Autodesk Inventor part; units mm, degrees
ref_plane "YZ Plane" through (0, 0, 0) normal (1, 0, 0) x (0, 1, 0)
ref_plane "XZ Plane" through (0, 0, 0) normal (0, 1, 0) x (-1, 0, 0)
ref_plane "XY Plane" through (0, 0, 0) normal (0, 0, 1) x (1, 0, 0)
sketch "Sketch1" plane through (0, 0, 0) normal (0, 1, 0) x (-1, 0, 0)
  line L0 (0, -7.0711) -> (0, -142.9289)
  line L1 (7.0711, 0) -> (142.9289, 0)
  line L2 (150, -7.0711) -> (150, -142.9289)
  line L3 (142.9289, -150) -> (7.0711, -150)
  line L4 (139.3934, -10.6066) -> (135.8579, -14.1421)
  line L5 (135.8579, -14.1421) -> (132.3223, -10.6066)
  line L6 (132.3223, -10.6066) -> (135.8579, -14.1421)
  line L7 (135.8579, -14.1421) -> (139.3934, -17.6777)
  line L8 (139.3934, -17.6777) -> (150, -7.0711)
  line L9 (132.3223, -10.6066) -> (142.9289, 0)
  line L10 (139.3934, -139.3934) -> (135.8579, -135.8579)
  line L11 (135.8579, -135.8579) -> (132.3223, -139.3934)
  line L12 (132.3223, -139.3934) -> (142.9289, -150)
  line L13 (135.8579, -135.8579) -> (139.3934, -132.3223)
  line L14 (139.3934, -132.3223) -> (150, -142.9289)
  line L15 (10.6066, -139.3934) -> (14.1421, -135.8579)
  line L16 (14.1421, -135.8579) -> (10.6066, -132.3223)
  line L17 (10.6066, -132.3223) -> (14.1421, -135.8579)
  line L18 (14.1421, -135.8579) -> (17.6777, -139.3934)
  line L19 (17.6777, -139.3934) -> (7.0711, -150)
  line L20 (10.6066, -132.3223) -> (0, -142.9289)
  line L21 (10.6066, -10.6066) -> (14.1421, -14.1421)
  line L22 (14.1421, -14.1421) -> (10.6066, -17.6777)
  line L23 (10.6066, -17.6777) -> (14.1421, -14.1421)
  line L24 (14.1421, -14.1421) -> (17.6777, -10.6066)
  line L25 (7.0711, 0) -> (17.6777, -10.6066)
  line L26 (10.6066, -17.6777) -> (0, -7.0711)
  line L27 (132.3223, -10.6066) -> (75, -67.9289)
  line L28 (67.9289, -75) -> (10.6066, -132.3223)
  line L29 (132.3223, -10.6066) -> (17.6777, -10.6066)
  line L30 (139.3934, -17.6777) -> (139.3934, -132.3223)
  line L31 (132.3223, -139.3934) -> (17.6777, -139.3934)
  line L32 (10.6066, -132.3223) -> (10.6066, -17.6777)
  line L33 (139.3934, -10.6066) -> (135.8579, -14.1421)
  line L34 (14.1421, -135.8579) -> (0, -150)
  line L35 (10.6066, -10.6066) -> (14.1421, -14.1421)
  line L36 (135.8579, -135.8579) -> (139.3934, -139.3934)
  line L37 (139.3934, -132.3223) -> (82.0711, -75)
  line L38 (75, -67.9289) -> (17.6777, -10.6066)
  line L39 (10.6066, -17.6777) -> (67.9289, -75)
  line L40 (75, -82.0711) -> (132.3223, -139.3934)
  line L41 (139.3934, -17.6777) -> (82.0711, -75)
  line L42 (75, -82.0711) -> (17.6777, -139.3934)
  point P0 (0, 0)
  dimension "d0" = 150
extrude "Extrusion1" add sketch "Sketch1" along normal blind 10 contours L26 L32 L20 L0 | L22 L24 L38 L27 L5 L7 L41 L37 L13 L11 L40 L42 L18 L16 L28 L39 | L25 L1 L9 L29 | L31 L12 L3 L19 | L8 L2 L14 L30
sketch "Sketch2" plane through (0, 10, 0) normal (0, 1, 0) x (1, 0, 0)
  line L0 (-17.6777, 10.6066) -> (-27.6777, 10.6066)
  line L1 (-17.6777, 10.6066) -> (-132.3223, 10.6066)
  line L2 (-27.6777, 10.6066) -> (-27.6777, 20.6066)
  line L3 (-75, 67.9289) -> (-17.6777, 10.6066)
  line L4 (-10.6066, 17.6777) -> (-67.9289, 75)
  line L5 (-20.6066, 27.6777) -> (-10.6066, 27.6777)
  line L6 (-10.6066, 27.6777) -> (-10.6066, 17.6777)
  line L7 (-10.6066, 132.3223) -> (-10.6066, 17.6777)
  line L8 (-132.3223, 10.6066) -> (-75, 67.9289)
  line L9 (-132.3223, 10.6066) -> (-122.3223, 10.6066)
  line L10 (-122.3223, 10.6066) -> (-122.3223, 20.6066)
  line L11 (-122.3223, 20.6066) -> (-129.3934, 27.6777)
  line L12 (-82.0711, 75) -> (-139.3934, 17.6777)
  line L13 (-139.3934, 27.6777) -> (-129.3934, 27.6777)
  line L14 (-139.3934, 17.6777) -> (-139.3934, 132.3223)
  line L15 (-139.3934, 27.6777) -> (-139.3934, 17.6777)
  line L16 (-139.3934, 17.6777) -> (-129.3934, 27.6777)
  line L17 (-132.3223, 10.6066) -> (-122.3223, 20.6066)
  line L18 (-139.3934, 132.3223) -> (-139.3934, 122.3223)
  line L19 (-139.3934, 122.3223) -> (-129.3934, 122.3223)
  line L20 (-139.3934, 132.3223) -> (-82.0711, 75)
  line L21 (-129.3934, 122.3223) -> (-122.3223, 129.3934)
  line L22 (-75, 82.0711) -> (-132.3223, 139.3934)
  line L23 (-122.3223, 129.3934) -> (-122.3223, 139.3934)
  line L24 (-132.3223, 139.3934) -> (-17.6777, 139.3934)
  line L25 (-122.3223, 139.3934) -> (-132.3223, 139.3934)
  line L26 (-17.6777, 139.3934) -> (-75, 82.0711)
  line L27 (-17.6777, 139.3934) -> (-27.6777, 139.3934)
  line L28 (-27.6777, 129.3934) -> (-27.6777, 139.3934)
  line L29 (-27.6777, 129.3934) -> (-20.6065, 122.3222)
  line L30 (-20.6065, 122.3222) -> (-10.6066, 122.3222)
  line L31 (-10.6066, 132.3223) -> (-20.6065, 122.3222)
  line L32 (-10.6066, 17.6777) -> (-20.6066, 27.6777)
  line L33 (-27.6777, 20.6066) -> (-17.6777, 10.6066)
  line L34 (-10.6066, 17.6777) -> (-10.6066, 27.6777)
  line L35 (-20.6066, 27.6777) -> (-10.6066, 17.6777)
  point P0 (0, 0)
  dimension "d9" = 10
  dimension "d10" = 10
  dimension "d11" = 10
extrude "Extrusion2" add sketch "Sketch2" against normal blind 10 contours L6 L4 L5 | L31 L7 L30 | L22 L24 L23 | L12 L14 L13 | L0 L2 L3 | L1 L8 L10 | L19 L14 L20 | L28 L24 L26
sketch "Sketch3" plane through (0, 10, 0) normal (0, 1, 0) x (1, 0, 0)
  line L0 (-67.9289, 75) -> (-10.6066, 132.3223)
  line L1 (-82.0711, 75) -> (-75, 67.9289)
  circle A0 centre (-75, 75) radius 1.25
  line L2 (-75, 82.0711) -> (-122.3223, 129.3934)
  line L3 (-82.0711, 75) -> (-129.3934, 27.6777)
  line L4 (-17.6777, 10.6066) -> (-10.6066, 17.6777)
  line L5 (-14.1421, 14.1421) -> (-17.6777, 10.6066)
  line L6 (-17.6777, 10.6066) -> (-14.1421, 14.1421)
  line L7 (-14.1421, 14.1421) -> (-17.6777, 10.6066)
  line L8 (-20.6066, 27.6777) -> (-67.9289, 75)
  line L9 (-10.6066, 132.3223) -> (-17.6777, 139.3934)
  circle A1 centre (-132.226, 17.774) radius 1.25
  circle A2 centre (-132.136, 132.136) radius 1.25
  circle A3 centre (-17.6777, 132.3223) radius 1.25
  circle A4 centre (-17.6777, 17.6777) radius 1.25
  point P0 (0, 0)
  dimension "d14" = 2.5
  dimension "d21" = 2.5
extrude "Extrusion3" add sketch "Sketch3" along normal blind 2.5
sketch "Sketch4" plane through (-10.6066, 0, -17.6777) normal (0.7071, 0, 0.7071) x (0.7071, 0, -0.7071)
  line L0 (-5, 0) -> (-5, 2.5)
  line L1 (-5, 2.5) -> (-2.5, 2.5)
  line L2 (-2.5, 2.5) -> (-2.5, 7.5)
  line L3 (-2.5, 7.5) -> (-7.5, 7.5)
  line L4 (-7.5, 7.5) -> (-7.5, 2.5)
  line L5 (-7.5, 2.5) -> (-5, 2.5)
  dimension "d25" = 2.5
  dimension "d26" = 2.5
  dimension "d27" = 5
  dimension "d28" = 5
extrude "Extrusion4" cut sketch "Sketch4" against normal blind 15
sketch "Sketch5" plane through (-132.3223, 0, -10.6066) normal (-0.7071, 0, 0.7071) x (0.7071, 0, 0.7071)
  line L0 (0, 0) -> (0, 10)
  line L1 (0, 0) -> (0, 5)
  line L2 (0, 5) -> (-2.5, 5)
  line L3 (-2.5, 5) -> (0, 5)
  line L4 (-2.5, 5) -> (-2.5, 7.5)
  line L5 (-2.5, 7.5) -> (-7.5, 7.5)
  line L6 (-7.5, 7.5) -> (-7.5, 2.5)
  line L7 (-7.5, 2.5) -> (-2.5, 2.5)
  line L8 (-2.5, 2.5) -> (-2.5, 5)
  point P0 (101.066, 0)
  dimension "d31" = 5
  dimension "d32" = 2.5
  dimension "d33" = 2.5
  dimension "d34" = 5
extrude "Extrusion5" cut sketch "Sketch5" against normal blind 15
sketch "Sketch6" plane through (-139.3934, 0, -132.3223) normal (-0.7071, 0, -0.7071) x (-0.7071, 0, 0.7071)
  line L0 (-5, 0) -> (-5, 2.5)
  line L1 (-7.5, 2.5) -> (-2.5, 2.5)
  line L2 (-5, 2.5) -> (-2.5, 2.5)
  line L3 (-2.5, 2.5) -> (-2.5, 7.5)
  line L4 (-2.5, 2.5) -> (-2.5, 7.5)
  line L5 (-2.5, 7.5) -> (-7.5, 7.5)
  line L6 (-2.5, 7.5) -> (-7.5, 7.5)
  line L7 (-7.5, 7.5) -> (-7.5, 2.5)
  line L8 (-7.5, 2.5) -> (-5, 2.5)
  dimension "d37" = 2.5
extrude "Extrusion6" cut sketch "Sketch6" against normal blind 15
sketch "Sketch7" plane through (-17.6777, 0, -139.3934) normal (0.7071, 0, -0.7071) x (-0.7071, 0, -0.7071)
  line L0 (0, 0) -> (-5, 0)
  line L1 (-10, 0) -> (0, 0)
  line L2 (-5, 0) -> (-5, 2.5)
  line L3 (-7.5, 2.5) -> (-2.5, 2.5)
  line L4 (-2.5, 2.5) -> (-2.5, 7.5)
  line L5 (-2.5, 2.5) -> (-2.5, 7.5)
  line L6 (-2.5, 7.5) -> (-7.5, 7.5)
  line L7 (-2.5, 7.5) -> (-7.5, 7.5)
  line L8 (-7.5, 7.5) -> (-7.5, 2.5)
  line L9 (-7.5, 7.5) -> (-7.5, 2.5)
  line L10 (-7.5, 2.5) -> (-5, 2.5)
  point P0 (-111.066, 0)
  dimension "d40" = 5
extrude "Extrusion7" cut sketch "Sketch7" against normal blind 15
sketch "Sketch8" plane through (0, 10, 0) normal (0, 1, 0) x (1, 0, 0)
  point P0 (0, 0)
properties part number "Frame"
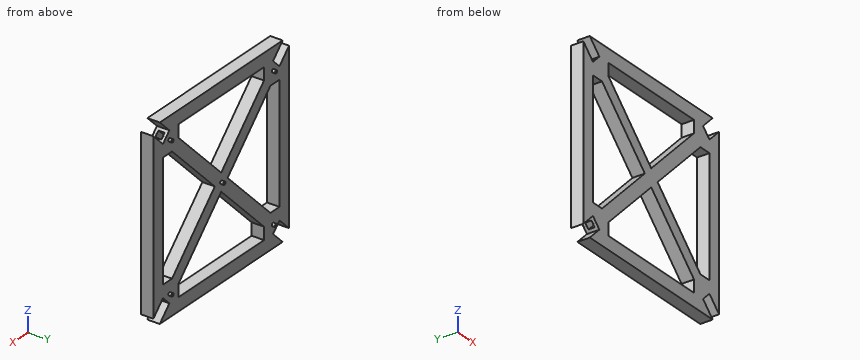
Can you work these out from the model? Positions are in its coordinate system, mm. Round coordinates to 2 decimals unless told otherwise and drop trailing zeros. Order: outer loops, then holes, each group sorted by start corner. A loop starts at its lowest first (then second) coordinate and runs counter-clockwise, first axis right, second up. Notation, with made-up numbers: (15.5, 17) -> (42.5, 17) arc R24 ccw to (42.5, 36) -> close; hole circle Ø5 at (0.5, 8.25). An arc over 180 degrees is marked (long way). Write each question's results on one line, items separated by ' | '. Start each with the question number.
Item 1: If we section it at B-B, the plane z = -120.5: Write out the boundary of the cut face in (x, y), then the cut area to 3 significant figures.
Item 2: Please list where these lines run through material, in increasing order: L1, parallel to Z at x = -46.5, y = 6; L2, parallel to X at y = 5.25, z = -112; L3, parallel to X at y = 5, z = -58.5.
Item 3: If we section it at A-A, the plane x = -113.5: Write out the boundary of the cut face in (y, z), then the cut area to 3 significant figures.
Item 4: Will these pins go through, and if not, where does the flat tip stop? pin 1 (4 mm diameter, centred on x = -17.5, z = -22.5, fed in from -Y); pin 2 (6 mm diameter, centred on x = -28, z = -18, fed in from +Y).
Results:
1) outline: (-150, 0) -> (-139.39, 0) -> (-139.39, 10) -> (-150, 10) -> close; (-127.57, 0) -> (-113.43, 0) -> (-113.43, 10) -> (-127.57, 10) -> close; (-36.57, 0) -> (-22.43, 0) -> (-22.43, 10) -> (-36.57, 10) -> close; (-10.61, 0) -> (0, 0) -> (0, 10) -> (-10.61, 10) -> close | area: 495 mm2
2) L1: z = -150 to -139.39, -110.57 to -96.43, -53.57 to -39.43, -10.61 to 0 | L2: x = -150 to -139.39, -119.07 to -104.93, -45.07 to -30.93, -10.61 to 0 | L3: x = -150 to -139.39, -98.57 to -84.43, -65.57 to -51.43, -10.61 to 0
3) outline: (0, -150) -> (10, -150) -> (10, -139.39) -> (0, -139.39) -> close; (0, -120.57) -> (10, -120.57) -> (10, -106.43) -> (0, -106.43) -> close; (0, -43.57) -> (10, -43.57) -> (10, -29.43) -> (0, -29.43) -> close; (0, -10.61) -> (10, -10.61) -> (10, 0) -> (0, 0) -> close | area: 495 mm2
4) pin 1: stops at y = 0 | pin 2: stops at y = 10
